```python
from build123d import *

# Parameters (mm, degrees)
SKETCH1_W           = 482.6
SKETCH1_H           = 52.578
BOSS_EXTRUDE1_DEPTH = 1308.608
FILLET1_R           = 25.1206
CUT_EXTRUDE1_DEPTH  = 483.6


with BuildPart() as part:
    # Sketch1 → Boss-Extrude1 (new body)
    with BuildSketch(Plane(origin=(0, 0, 0), x_dir=(1, 0, 0), z_dir=(0, 1, 0))):
        Rectangle(SKETCH1_W, SKETCH1_H)
    extrude(amount=BOSS_EXTRUDE1_DEPTH)

    # Fillet1
    fillet1_edges = [part.edges().sort_by_distance(p)[0] for p in [
        (0, 1308.608, -26.289),
        (0, 0, -26.289),
        (0, 0, 26.289),
        (0, 1308.608, 26.289),
    ]]
    fillet(fillet1_edges, radius=FILLET1_R)

    # Sketch2 → Cut-Extrude1 (cut, through all)
    with BuildSketch(Plane(origin=(241.3, 0, 0), x_dir=(0, 0, -1), z_dir=(1, 0, 0))):
        with BuildLine():
            Line((24.9428, 25.1206), (24.9428, 1283.4874))
            ThreePointArc((24.9428, 1283.4874), (17.979439459, 1300.298439459), (1.1684, 1307.2618))
            Line((1.1684, 1307.2618), (-1.1684, 1307.2618))
            ThreePointArc((-1.1684, 1307.2618), (-17.979439459, 1300.298439459), (-24.9428, 1283.4874))
            Line((-24.9428, 1283.4874), (-24.9428, 25.1206))
            ThreePointArc((-24.9428, 25.1206), (-17.979439459, 8.309560541), (-1.1684, 1.3462))
            Line((-1.1684, 1.3462), (1.1684, 1.3462))
            ThreePointArc((1.1684, 1.3462), (17.979439459, 8.309560541), (24.9428, 25.1206))
        make_face()
    extrude(amount=-CUT_EXTRUDE1_DEPTH, mode=Mode.SUBTRACT)


solid = part.part
```
Geometry: final body of the model. Coordinates: model frame, mm. A direction names the side the tool comes from. Round coordinates to 2 decimals unless told otherwise and drop trailing zeros. Loops run counter-clockwise (first coordinate to the right, second up) from the corner with the lowest first, then second, coordinate; pieces in that order, holes last. Notation, with made-up numbers: (-29.5, 7) -> (2.5, 7) arc R29 cw to (2.5, 33) -> close; hole circle Ø3 at (86, 48.25). An arc over 180 degrees is marked (long way). Write each question's results on one line, items separated by ' | '.
Item 1: Line query: probe 1 along Z at (x, y) = (-163, 1192); probe 2 along Y at (x, z) = (-86.5, -2.5); probe 3 along Y at (x, z) = (-147, -13). Output: solid intervals per line, ascending. Write a range as [from, to].
Answers below:
probe 1: z = [-26.29, -24.94], [24.94, 26.29] | probe 2: y = [0.04, 1.38], [1307.22, 1308.57] | probe 3: y = [2.96, 4.5], [1304.11, 1305.65]
Item 2: Pull-direction query (Y, two-part tool) for faces 3 (the face through (3.378, 7.554, 19.126)), 4 (the face through (3.378, 1300.482, 17.794)), 5 (the face through (3.38, 1301.05, 19.13)); classes: pulls with the +Y half, pulls with the -Y half, needs draft (parallel to the pull), parting line crosses it, or undercut.
Answers below:
face 3: pulls with the -Y half | face 4: undercut | face 5: pulls with the +Y half
Item 3: Pin query (flat end, axial travel): pin 1 Ø6 at (x, z) = (28, -17.5) entering from -Y; pin 2 Ø1.5 at (x, z) = (-185, -19) entering from -Y; pin 3 Ø4 at (x, z) = (-71.5, 20) entering from -Y. Return the tip coordinate at first contact, or that it passes through.
Answers below:
pin 1: stops at y = 3.83 | pin 2: stops at y = 6.7 | pin 3: stops at y = 6.47
Item 4: Cut plane B-B on x = 212. Return the cut outline in (y, z), and give its area (3 significant figures).
Answers below:
outline: (0, -1.17) arc R25.12 ccw to (25.12, -26.29) -> (1283.49, -26.29) arc R25.12 ccw to (1308.61, -1.17) -> (1308.61, 1.17) arc R25.12 ccw to (1283.49, 26.29) -> (25.12, 26.29) arc R25.12 ccw to (0, 1.17) -> close; hole (1.35, -1.17) arc R23.77 ccw to (25.12, -24.94) -> (1283.49, -24.94) arc R23.77 ccw to (1307.26, -1.17) -> (1307.26, 1.17) arc R23.77 ccw to (1283.49, 24.94) -> (25.12, 24.94) arc R23.77 ccw to (1.35, 1.17) -> close | area: 3,600 mm²
Item 5: Cut plane A-A on y = 497. Return the cut outline in (x, z), and give its area (3 significant figures).
Answers below:
outline: (-241.3, -26.29) -> (241.3, -26.29) -> (241.3, -24.94) -> (-241.3, -24.94) -> close; (-241.3, 24.94) -> (241.3, 24.94) -> (241.3, 26.29) -> (-241.3, 26.29) -> close | area: 1,300 mm²
Item 6: Set-up query: faces 1 (the face through (3.378, 1300.113, -18.163)), 2 (the face through (3.38, 1301.05, -19.13)). Return all of +Z, -Z, +X, -X, +Y, -Y with unobstructed straight access to the full face (end or side cutting, diameter ignored); none if empty.
Answers below:
face 1: +X, -X | face 2: -Z, +X, -X, +Y
Item 7: Cut plane C-C on z = -17. Return the cut outline in (x, y).
Answers below:
outline: (-241.3, 5.62) -> (241.3, 5.62) -> (241.3, 7.38) -> (-241.3, 7.38) -> close; (-241.3, 1301.22) -> (241.3, 1301.22) -> (241.3, 1302.99) -> (-241.3, 1302.99) -> close
